Read the model definition and answer for the solid it produces. Units are mm, in the model's axes. Coordinates: 2 decimals unless noted, no trailing zeros. Loops run counter-clockwise (first coordinate to the right, second up) from the corner with the lowest first, then second, coordinate; pieces in that order, holes last. Notation, with made-up numbers: (72, 54) -> (94, 54) arc R11 cw to (94, 67) -> close; hole circle Ø5 at (-23.5, 67). An arc over 180 degrees is marked (long way). One line per question, with ' | ' between items. Start each with the question number.
Autodesk Inventor part; units mm, degrees
ref_plane "YZ Plane" through (0, 0, 0) normal (1, 0, 0) x (0, 1, 0)
ref_plane "XZ Plane" through (0, 0, 0) normal (0, 1, 0) x (-1, 0, 0)
ref_plane "XY Plane" through (0, 0, 0) normal (0, 0, 1) x (1, 0, 0)
sketch "Sketch1" plane through (0, 0, 0) normal (0, 0, 1) x (1, 0, 0)
  circle A0 centre (0, 0) radius 5.7
  dimension "d0" = 11.4
extrude "Extrusion1" add sketch "Sketch1" along normal blind 2
chamfer "Chamfer1" distance 0.8 angle 45 1 edges at (-5.7, 0, 2)
sketch "Sketch2" plane through (0, 0, 0) normal (0, 0, 1) x (1, 0, 0)
  circle A0 centre (0, 0) radius 2.9
  dimension "d6" = 5.8
extrude "Extrusion2" cut sketch "Sketch2" along normal up to surface (2 mm away)
properties part number "Insert2mm"
(1) Determine the mould class of faces 1 (the cylindrical face through (-2.9, -0.1, 1)), 2 (the flat face through (-0.1, -3.2, 2)), 3 (the cylindrical face through (-4.5, 3.5, 0.6)) for opening direction X: +X half, -X half, draft (parallel to the pull), parting line (faces both ways), or undercut.
(2) Find the intervals of material crossed by probe 1 along Y at (x, z) = (0, 0.65); probe 2 along X at (y, z) = (-0.25, 1.5); probe 3 along X at (y, z) = (1, 0.75), in increasing order. Write a range as from..to.
(3) Section D-D on z = 0.45 is taken. Write down the section's boundary in (x, y), plus the area to 3 significant figures.
(4) Section A-A on x = 0 is taken. Write down the section's boundary in (y, z), plus the area to 3 significant figures.
(5) This flat-tipped pin is pushed along its axis until it touches: pin 1 Ø1 at (x, z) = (2, 0.5) entering from -Y. Where does it stop, or does it pass through?
(6) Section C-C on z = 1.45 is taken. Write down the section's boundary in (x, y), plus the area to 3 significant figures.
Working result:
1) face 1: undercut | face 2: draft | face 3: parting line
2) probe 1: y = -5.7..-2.9, 2.9..5.7 | probe 2: x = -5.39..-2.89, 2.89..5.39 | probe 3: x = -5.61..-2.72, 2.72..5.61
3) outline: circle Ø11.4 at (0, 0); hole circle Ø5.8 at (0, 0) | area: 75.6 mm2
4) outline: (-5.7, 0) -> (-2.9, 0) -> (-2.9, 2) -> (-4.9, 2) -> (-5.7, 1.2) -> close; (2.9, 0) -> (5.7, 0) -> (5.7, 1.2) -> (4.9, 2) -> (2.9, 2) -> close | area: 10.6 mm2
5) pin 1: stops at y = -5.5
6) outline: circle Ø10.9 at (0, 0); hole circle Ø5.8 at (0, 0) | area: 66.9 mm2
